from build123d import *

# Parameters (mm, degrees)
ESQUISSE1_W             = 10.9
ESQUISSE1_H             = 8
ESQUISSE1_W_2           = 2.35
ESQUISSE1_H_2           = 2.85
BOSS_EXTRU_1_DEPTH      = 19.49
CHANFREIN1_SIZE         = 2
ESQUISSE2_W             = 15.6
ESQUISSE2_H             = 4
ENL_V_MAT_EXTRU_1_DEPTH = 10
CONG_1_R                = 1


with BuildPart() as part:
    # Esquisse1 → Boss.-Extru.1 (new body)
    with BuildSketch(Plane(origin=(0, 0, 0), x_dir=(1, 0, 0), z_dir=(0, 1, 0))):
        with Locations((5.45, 4)):
            Rectangle(ESQUISSE1_W, ESQUISSE1_H)
        with Locations((-1.175, 4)):
            Rectangle(ESQUISSE1_W_2, ESQUISSE1_H_2)
        with Locations((12.075, 4)):
            Rectangle(ESQUISSE1_W_2, ESQUISSE1_H_2)
    extrude(amount=BOSS_EXTRU_1_DEPTH)

    # Chanfrein1
    chanfrein1_edges = [part.edges().sort_by_distance(p)[0] for p in [
        (5.45, 0, 0),
    ]]
    chamfer(chanfrein1_edges, length=CHANFREIN1_SIZE)

    # Esquisse2 → Enlèv. mat.-Extru.1 (cut)
    with BuildSketch(Plane(origin=(0, 19.49, 0), x_dir=(1, 0, 0), z_dir=(0, 1, 0))):
        with Locations((5.45, 6)):
            Rectangle(ESQUISSE2_W, ESQUISSE2_H)
    extrude(amount=-ENL_V_MAT_EXTRU_1_DEPTH, mode=Mode.SUBTRACT)

    # Congé1
    cong_1_edges = [part.edges().sort_by_distance(p)[0] for p in [
        (-2.35, 9.745, -2.575),
        (13.25, 9.745, -2.575),
        (-2.35, 4.745, -5.425),
        (13.25, 4.745, -5.425),
    ]]
    fillet(cong_1_edges, radius=CONG_1_R)


solid = part.part
Design review of the part built by this model. Coordinates are the model's own, in mm. A direction names the side the tool comes from. Coordinates: 2 decimals unless noted, no trailing zeros. Loops run counter-clockwise (first coordinate to the right, second up) from the corner with the lowest first, then second, coordinate; pieces in that order, holes last. Notation, with made-up numbers: (29.5, 60.25) - (36.5, 60.25) arc R30 cw to (36.5, 87.25) - close; hole circle Ø7 at (-14.5, 78). An arc over 180 degrees is marked (long way). Use CSV: the item, a comma, the result in double quotes. Start each with the question number.
1. Add section B-B on x = 2. Give the boundary of the cut face in (y, z), plus the area to 3 significant figures.
2. For faces 4 (the flat face through (0, 5, -7)), 5 (the flat face through (10.9, 10, -1)), 6 (the flat face through (12, 5, -5.425)), list the 3-axis set-ups (+Z, -Z, +X, -X, +Y, -Y) from which the entire face can be reached by the end or side of a thin tool; tool diameter is ignored.
3. To check wall thickness, follow probe 1 along X at (y, z) = (10.25, -1.5); probe 2 along Z at (x, y) = (11.25, 17.5) (3 decimals); probe 3 along Y at (x, z) = (-0.75, -4.5). State the ranges of each line that lie inside material, in increasing order.
4. Add section A-A on y = 14.75. Give the boundary of the cut face in (x, z) (3 decimals).
5. Mouldability with a two-part tool opening along X and no side actions: class faces 1 (the flat face through (-2.35, 7, -4)), 2 (the flat face through (-1, 5, -5.425)), 3 (the cylindrical face through (12.965, 4.811, -5.124)) as released by +X, released by -X, zero draft, split by the parting line, or undercut.
6. Add section C-C on z = -1.75. Give the boundary of the cut face in (x, y), plus the area to 3 significant figures.
7. Clearance check with flat-ended pins moving along their axes: pin 1 (3 mm diameter, centred on y = 6.5, z = -6.5, fed in from +X); pin 2 (3 mm diameter, centred on y = 10, z = -1, fed in from -X); pin 3 (1.1 mm diameter, centred on x = 12, y = 7, fed in from -Z) (3 decimals); pin 4 (2 mm diameter, centred on x = 1.5, z = -7, fed in from -Y). State where each tip first meets the part, or that it passes through.
8. Add section D-D on y = 7.75. Give the boundary of the cut face in (x, z) (3 decimals).
Resolved:
1,outline,"(0, -8) - (9.49, -8) - (9.49, -4) - (19.49, -4) - (19.49, 0) - (2, 0) - (0, -2) - close"
1,area,"114 mm2"
2,face 4,"-Z, -X, +Y, -Y"
2,face 5,"+Z, +X, +Y, -Y"
2,face 6,"-Z, +X, +Y, -Y"
3,probe 1,"0 to 10.9"
3,probe 2,"-4 to -2.575"
3,probe 3,"0 to 9.49"
4,outline,"(-2.35, -4) - (13.25, -4) - (13.25, -3.575) arc R1 ccw to (12.25, -2.575) - (10.9, -2.575) - (10.9, 0) - (0, 0) - (0, -2.575) - (-1.35, -2.575) arc R1 ccw to (-2.35, -3.575) - close"
5,face 1,"released by -X"
5,face 2,"zero draft"
5,face 3,"released by +X"
6,outline,"(0, 0.25) - (10.9, 0.25) - (10.9, 19.49) - (0, 19.49) - close"
6,area,"210 mm2"
7,pin 1,"x = 13.07"
7,pin 2,"x = 0"
7,pin 3,"z = -5.425"
7,pin 4,"y = 0"
8,outline,"(-2.35, -4.425) arc R1 ccw to (-1.35, -5.425) - (0, -5.425) - (0, -8) - (10.9, -8) - (10.9, -5.425) - (12.25, -5.425) arc R1 ccw to (13.25, -4.425) - (13.25, -3.575) arc R1 ccw to (12.25, -2.575) - (10.9, -2.575) - (10.9, 0) - (0, 0) - (0, -2.575) - (-1.35, -2.575) arc R1 ccw to (-2.35, -3.575) - close"
